Design review of the part built by this model. Coordinates are the model's own, in mm. Face numbers are marked on the shaded views. A direction names the side the tool comes from. Give positions to 0.01 mm unless a question says otherwise; leave off trailing zeros. Order: outer loops, then holes, each group sorted by start corner. A loop starts at its lowest first (then second) coordinate and runs counter-clockwise, first axis right, second up. Notation, with made-up numbers: (49.5, -18) -> (65.5, -18) arc R31 ccw to (65.5, 19) -> close; hole circle Ø3 at (20.5, 8). An arc over 180 degrees is marked (long way). One line per item, written item: value. Start each with the question number.
1) Wall thickness on line 1 along X through (y, z) = (-13, 114); line 2 along Z through (x, y) = (50.8, -14.4); line 3 along Z through (x, y) = (50, -14): over which ranges is each line inside the solid? List them lowest first. Write a range as from..to.
2) Consider section A-A (x = 22). State the section outline as (y, z) points, plus the area to 3 significant figures.
3) The part is to be moulded in two halves that separate along X. For the marked faces 4 and 5, say which applies: released by +X, released by -X, zero draft, split by the parting line, or undercut.
4) For pin 1 (4 mm diameter, centred on x = 49, z = 114, fed in from -Y); pin 2 (1 mm diameter, centred on x = 58, z = 43, fed in from -Y); pin 3 (10.5 mm diameter, centred on x = 38.5, z = 135, fed in from -Y), all flat-tipped, find the tip position at first contact; note any pin that passes through.
5) Tool access review of the marked faces 1, 2 and 3: name each direction out of +Z, -Z, +X, -X, +Y, -Y from which nothing blocks a thin tool from reaching the whole face with its end or side.
6) Consider section B-B (y = 21). State the section outline as (x, z) points, plus the area to 3 significant figures.
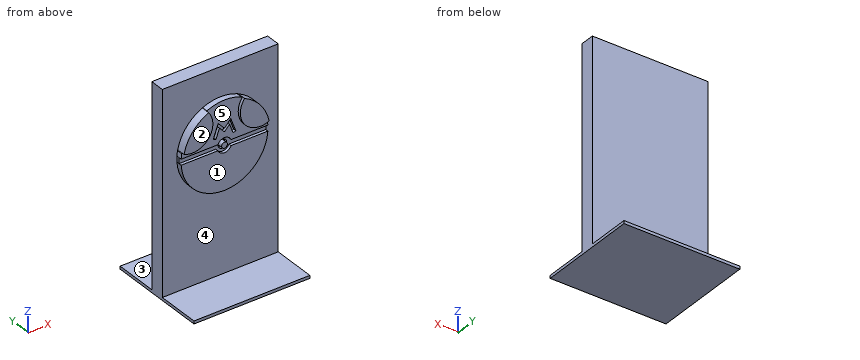
from build123d import *

# Parameters (mm, degrees)
F0_W          = 101.6
F0_H          = 175.26
F1_DEPTH      = 12.7
F0_H_2        = 2.54
F2_DEPTH      = 50.8
F2_DEPTH_BACK = 38.1
F4_DEPTH      = 7.62
F3_R          = 2.54
F5_DEPTH      = 5.08
F3_R_2        = 3.81
F6_DEPTH      = 2.54


with BuildPart() as f1:
    # F0 (on Front) → F1 (new body)
    with BuildSketch(Plane.XZ):
        with Locations((50.8, 90.17)):
            Rectangle(F0_W, F0_H)
    extrude(amount=F1_DEPTH)

    # F0 (on Front) → F2 (join, two sides)
    with BuildSketch(Plane.XZ) as f2_sk:
        with Locations((50.8, 1.27)):
            Rectangle(F0_W, F0_H_2)
    extrude(amount=F2_DEPTH)
    extrude(f2_sk.sketch, amount=-F2_DEPTH_BACK)

    # F3 (on face) → F4 (join)
    with BuildSketch(Plane.XZ.offset(12.7)):
        with BuildLine():
            ThreePointArc((66.593426, 148.972434), (66.697351, 126.95609), (88.130224, 121.92))
            ThreePointArc((88.130224, 121.92), (80.607534, 138.030169), (66.593426, 148.972434))
        make_face()
        with BuildLine():
            ThreePointArc((13.469776, 121.92), (34.902649, 126.95609), (35.006574, 148.972434))
            ThreePointArc((35.006574, 148.972434), (20.992466, 138.030169), (13.469776, 121.92))
        make_face()
    extrude(amount=F4_DEPTH)

    # F3 (on face) → F5 (join)
    with BuildSketch(Plane.XZ.offset(12.7)):
        with BuildLine():
            ThreePointArc((12.784761, 111.76), (50.8, 76.2), (88.815239, 111.76))
            Line((88.815239, 111.76), (56.619871, 111.76))
            ThreePointArc((56.619871, 111.76), (50.8, 107.95), (44.980129, 111.76))
            Line((44.980129, 111.76), (12.784761, 111.76))
        make_face()
        with BuildLine():
            Line((56.619871, 116.84), (88.815239, 116.84))
            ThreePointArc((88.815239, 116.84), (88.5956, 119.106519), (88.24095, 121.355868))
            ThreePointArc((88.24095, 121.355868), (88.186651, 121.638143), (88.130224, 121.92))
            ThreePointArc((88.130224, 121.92), (66.697351, 126.95609), (66.593426, 148.972434))
            ThreePointArc((66.593426, 148.972434), (66.013621, 149.230727), (65.429595, 149.479326))
            ThreePointArc((65.429595, 149.479326), (50.361762, 152.39748), (35.365042, 149.133491))
            ThreePointArc((35.365042, 149.133491), (35.1856, 149.053425), (35.006574, 148.972434))
            ThreePointArc((35.006574, 148.972434), (34.902649, 126.95609), (13.469776, 121.92))
            ThreePointArc((13.469776, 121.92), (13.390944, 121.523058), (13.316333, 121.125301))
            ThreePointArc((13.316333, 121.125301), (12.989788, 118.990187), (12.784761, 116.84))
            Line((12.784761, 116.84), (44.980129, 116.84))
            ThreePointArc((44.980129, 116.84), (50.8, 120.65), (56.619871, 116.84))
        make_face()
        Polygon((43.324096, 121.942925), (40.894, 122.682), (45.237656, 134.616096), (50.8, 128.524), (56.362344, 134.616096), (60.706, 122.682), (58.275904, 121.942925), (55.235345, 130.296792), (50.8, 125.476), (46.364655, 130.296792), align=None, mode=Mode.SUBTRACT)
        with Locations((50.8, 114.3)):
            Circle(F3_R)
    extrude(amount=F5_DEPTH)

    # F3 (on face) → F6 (join)
    with BuildSketch(Plane.XZ.offset(12.7)):
        with BuildLine():
            ThreePointArc((12.784761, 116.84), (12.7, 114.3), (12.784761, 111.76))
            Line((12.784761, 111.76), (44.980129, 111.76))
            ThreePointArc((44.980129, 111.76), (44.45, 114.3), (44.980129, 116.84))
            Line((44.980129, 116.84), (12.784761, 116.84))
        make_face()
        with BuildLine():
            ThreePointArc((57.15, 114.3), (57.016055, 115.597366), (56.619871, 116.84))
            ThreePointArc((56.619871, 116.84), (50.8, 120.65), (44.980129, 116.84))
            ThreePointArc((44.980129, 116.84), (44.45, 114.3), (44.980129, 111.76))
            ThreePointArc((44.980129, 111.76), (50.8, 107.95), (56.619871, 111.76))
            ThreePointArc((56.619871, 111.76), (57.016055, 113.002634), (57.15, 114.3))
        make_face()
        with Locations((50.8, 114.3)):
            Circle(F3_R_2, mode=Mode.SUBTRACT)
        with BuildLine():
            ThreePointArc((88.815239, 111.76), (88.878804, 113.029293), (88.9, 114.3))
            ThreePointArc((88.9, 114.3), (88.878804, 115.570707), (88.815239, 116.84))
            Line((88.815239, 116.84), (56.619871, 116.84))
            ThreePointArc((56.619871, 116.84), (57.016055, 115.597366), (57.15, 114.3))
            ThreePointArc((57.15, 114.3), (57.016055, 113.002634), (56.619871, 111.76))
            Line((56.619871, 111.76), (88.815239, 111.76))
        make_face()
        Polygon((45.237656, 134.616096), (40.894, 122.682), (43.324096, 121.942925), (46.364655, 130.296792), (50.8, 125.476), (55.235345, 130.296792), (58.275904, 121.942925), (60.706, 122.682), (56.362344, 134.616096), (50.8, 128.524), align=None)
    extrude(amount=F6_DEPTH)


solid = f1.part
Checked values:
1. line 1: x = 12.7..47, 48.28..53.32, 54.6..88.9
1. line 2: z = 0..2.54, 76.2..110.49, 111.76..116.84, 118.11..152.4
1. line 3: z = 0..2.54, 76.21..110.57, 111.89..116.71, 118.03..152.39
2. outline: (-50.8, 0) -> (38.1, 0) -> (38.1, 2.54) -> (0, 2.54) -> (0, 177.8) -> (-12.7, 177.8) -> (-12.7, 139.24) -> (-20.32, 139.24) -> (-20.32, 120.28) -> (-17.78, 120.28) -> (-17.78, 116.84) -> (-15.24, 116.84) -> (-15.24, 111.76) -> (-17.78, 111.76) -> (-17.78, 89.36) -> (-12.7, 89.36) -> (-12.7, 2.54) -> (-50.8, 2.54) -> close
2. area: 2,740 mm^2
3. face 4: zero draft
3. face 5: undercut
4. pin 1: stops at y = -17.78
4. pin 2: stops at y = -12.7
4. pin 3: stops at y = -20.32
5. face 1: +X, -X, -Y
5. face 2: +Z, +X, -X, -Y
5. face 3: +Z, +X, -X, +Y
6. outline: (0, 0) -> (101.6, 0) -> (101.6, 2.54) -> (0, 2.54) -> close
6. area: 258 mm^2
